Geometry check sheet. Reference: the model listing, model coordinates, mm. Face numbers are marked on the shaded views. A direction names the side the tool comes from. Coordinates: 2 decimals unless noted, no trailing zeros. Order: outer loops, then holes, each group sorted by start corner. A loop starts at its lowest first (then second) coordinate and runs counter-clockwise, first axis right, second up. Notation, with made-up numbers: (70.5, 4.25) - (101.5, 4.25) arc R19 ccw to (101.5, 41.25) - close; hole circle Ø7 at (66, 3). An arc over 180 degrees is marked (long way). One line per item, written item: value. Start each with the question number.
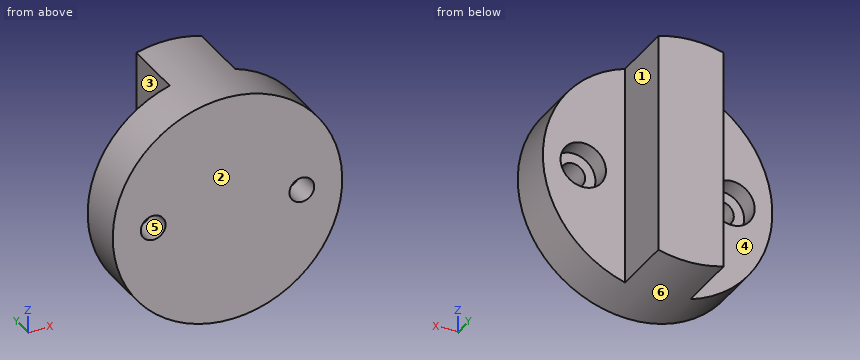
```python
from build123d import *

# Parameters (mm, degrees)
SKETCH1_R                      = 11.1125
BOSS_EXTRUDE1_DEPTH            = 11.1125
CUT_EXTRUDE1_START             = -6.35
CUT_EXTRUDE1_DEPTH             = 6.35
CBORE_FOR_M2_SHCS1_D           = 2.4
CBORE_FOR_M2_SHCS1_CBORE_D     = 4.4
CBORE_FOR_M2_SHCS1_CBORE_DEPTH = 2


with BuildPart() as part:
    # Sketch1 → Boss-Extrude1 (new body)
    with BuildSketch(Plane(origin=(0, 0, 0), x_dir=(1, 0, 0), z_dir=(0, 1, 0))):
        with Locations(Location((0, 0, 0), (0, 0, 270))):
            Circle(SKETCH1_R)
    extrude(amount=BOSS_EXTRUDE1_DEPTH)

    # Sketch2 → Cut-Extrude1 (cut)
    with BuildSketch(Plane(origin=(0, 11.1125, 0), x_dir=(1, 0, 0), z_dir=(0, 1, 0)).offset(CUT_EXTRUDE1_START)):
        with BuildLine():
            Line((-3.1623, 10.653051908), (-3.1623, -10.653051908))
            ThreePointArc((-3.1623, -10.653051908), (-11.1125, 0), (-3.1623, 10.653051908))
        make_face()
        with BuildLine():
            Line((3.1623, 10.653051908), (3.1623, -10.653051908))
            ThreePointArc((3.1623, -10.653051908), (11.1125, 0), (3.1623, 10.653051908))
        make_face()
    extrude(amount=CUT_EXTRUDE1_DEPTH, mode=Mode.SUBTRACT)

    # CBORE for M2 SHCS1 (through all)
    with Locations(Plane(origin=(0, 4.7625, 0), x_dir=(1, 0, 0), z_dir=(0, 1, 0))):
        with Locations((-7.2, 0), (7.2, 0)):
            CounterBoreHole(CBORE_FOR_M2_SHCS1_D / 2, CBORE_FOR_M2_SHCS1_CBORE_D / 2, CBORE_FOR_M2_SHCS1_CBORE_DEPTH)


solid = part.part
```
Q1. Cross-section at A-A, the plane z = 0. Enter the section's corners in (x, y), and give its area (3 significant figures).
Q2. Material ranges on probe 1 along X at (y, z) = (3, -0.25); probe 2 along X at (y, z) = (10.5, 1.75); probe 3 along Z at (x, y) = (-7.2, 4.05), recorded low to high.
Q3. Set-up check for the marked faces 1, 2 and 3: record each of +Z, -Z, +X, -X, +Y, -Y from which the full face is reachable in a straight line by a thin tool's end or side.
Q4. Cross-section at B-B, the plane x = 7.2. Enter the section's corners in (y, z), and give its area (3 significant figures).
Q5. Gauge pin test, flat ends, axial feed: P1, Ø1.4, axis at x = -7.2, z = 0, coming from the -Y side (3 decimals); P2, Ø1, axis at x = 1, y = 8, coming from the +Z side; P3, Ø3, axis at x = 7.2, z = 0, coming from the -Y side; P4, Ø8.5, axis at x = -8, z = 5, coming from the +Y side. Record the tip position at first contact, or that the pin passes through.
Q6. Cross-section at C-C, the plane y = 1.75. Enter the section's corners in (x, z) (1 decimal).
Q7. Release check for a two-part mould opening along Z. For the marked faces 4, 5 and 6 record: released by +Z, released by -Z, zero draft, split by the parting line, or undercut.
Q8. Cross-section at D-D, the plane z = -5.5. Enter the section's corners in (x, y), and give its area (3 significant figures).
Check result:
1. outline: (-11.11, 0) - (-8.4, 0) - (-8.4, 2.76) - (-9.4, 2.76) - (-9.4, 4.76) - (-11.11, 4.76) - close; (-6, 0) - (6, 0) - (6, 2.76) - (5, 2.76) - (5, 4.76) - (3.16, 4.76) - (3.16, 11.11) - (-3.16, 11.11) - (-3.16, 4.76) - (-5, 4.76) - (-5, 2.76) - (-6, 2.76) - close; (8.4, 0) - (11.11, 0) - (11.11, 4.76) - (9.4, 4.76) - (9.4, 2.76) - (8.4, 2.76) - close
1. area: 115 mm2
2. probe 1: x = -11.11 to -9.39, -5.01 to 5.01, 9.39 to 11.11
2. probe 2: x = -3.16 to 3.16
2. probe 3: z = -8.46 to -2.2, 2.2 to 8.46
3. face 1: +Z, -Z, +X, +Y
3. face 2: +Z, -Z, +X, -X, -Y
3. face 3: +Z, -Z, -X, +Y
4. outline: (0, -8.46) - (4.76, -8.46) - (4.76, -2.2) - (2.76, -2.2) - (2.76, -1.2) - (0, -1.2) - close; (0, 1.2) - (2.76, 1.2) - (2.76, 2.2) - (4.76, 2.2) - (4.76, 8.46) - (0, 8.46) - close
4. area: 65.2 mm2
5. P1: passes through
5. P2: stops at z = 11.1
5. P3: stops at y = 0
5. P4: stops at y = 4.76
6. outline: circle Ø22.2 at (0, 0); hole circle Ø2.4 at (-7.2, 0); hole circle Ø2.4 at (7.2, 0)
7. face 4: zero draft
7. face 5: undercut
7. face 6: split by the parting line
8. outline: (-9.66, 0) - (9.66, 0) - (9.66, 4.76) - (3.16, 4.76) - (3.16, 11.11) - (-3.16, 11.11) - (-3.16, 4.76) - (-9.66, 4.76) - close
8. area: 132 mm2
